Could you check a few things on this model? Use its own coordinates, in mm. Face numbers are marked on the shaded views. A direction names the side the tool comes from. Coordinates: 2 decimals unless noted, no trailing zeros. Order: outer loops, then holes, each group sorted by start corner. A loop starts at its lowest first (then second) coordinate and runs counter-clockwise, first axis right, second up. Notation, with made-up numbers: (-7, 12.25) - (30, 12.25) arc R18 ccw to (30, 26.25) - close; hole circle Ø2 at (-34, 35.5). An arc over 180 degrees is marked (long way). Answer as a JSON object with one key per item and string values. Group by question number.
(1) Which directions (+Z, -Z, +X, -X, +Y, -Y) give clear straight access to the entire face, cutting with the end or side of a thin tool? Please do the marked faces 4, 5 and 6.
(2) Imagine slicing it at B-B, the plane z = -7. Give the number of separate pieces and of enclosed holes in the cut face, and give its area (3 significant figures).
(3) We'd pull the mould along Y, two halves only. Please class the marked faces 1, 2 and 3: pulls with the +Y half, pulls with the -Y half, needs draft (parallel to the pull), parting line crosses it, or undercut.
(4) Please list where these lines run through material, in increasing order: probe 1 along Z at (x, y) = (22, -7); probe 2 along Y at (x, z) = (3.5, -21); probe 3 along Z at (x, y) = (3.5, -31).
(5) Will these pins go through, and if not, where does the flat tip stop? P1, Ø4, axis at y = -43, z = -8, coming from the -X side; P2, Ø5, axis at x = 13.5, z = -18.5, coming from the +Y side; P3, Ø2, axis at x = 0.5, y = -44.5, coming from the -Z side.
(6) Imagine slicing it at A-A, the plane z = -25. Write out the boundary of the cut face in (x, y).
from build123d import *

# Parameters (mm, degrees)
F1_DEPTH  = 17.5
F1_TAPER  = -3.5
F3_DEPTH  = 75
F4_T      = 2
F5_W      = 12.5
F5_H      = 3.5
F6_DEPTH  = 17.5010001
F7_R      = 4
F8_DEPTH  = 31.5
F9_SIZE   = 3
F11_W     = 25
F11_H     = 20
F12_DEPTH = 10


# Not quite as in the source:
# - a shell that OpenCascade refuses in one call is made with other operations: the cavity is built on its own and cut out


with BuildPart() as f1:
    # F0 (on Top) → F1 (new body)
    with BuildSketch(Plane.XY):
        with BuildLine():
            Line((-40.5, -45), (40.5, -45))
            ThreePointArc((40.5, -45), (41.9142135624, -44.4142135624), (42.5, -43))
            Line((42.5, -43), (42.5, 43))
            ThreePointArc((42.5, 43), (41.9142135624, 44.4142135624), (40.5, 45))
            Line((40.5, 45), (-40.5, 45))
            ThreePointArc((-40.5, 45), (-41.9142135624, 44.4142135624), (-42.5, 43))
            Line((-42.5, 43), (-42.5, -43))
            ThreePointArc((-42.5, -43), (-41.9142135624, -44.4142135624), (-40.5, -45))
        make_face()
    extrude(amount=-F1_DEPTH, taper=F1_TAPER)

    # F2 (on Front) → F3 (cut, symmetric)
    with BuildSketch(Plane.XZ):
        Polygon((-20, -17.5), (0, -17.5), (20, -17.5), (12, -9.5), (0, -9.5), (-12, -9.5), align=None)
    extrude(amount=F3_DEPTH, both=True, mode=Mode.SUBTRACT)

    # F4: shell of thickness 2, made by hand


with BuildPart() as f4_core1:
    # F4_t2: copy of F1
    add(f1.part)

    # the walls: a layer under each face that stays
    f4_faces = [f4_core1.faces().sort_by_distance(p)[0] for p in [
        (0, -45.5351729263, -8.75),
        (-42.2926379677, -44.7926379677, -8.75),
        (42.2926379677, -44.7926379677, -8.75),
        (0, 0, 0),
        (-43.0351729263, 0, -8.75),
        (-42.2926379677, 44.7926379677, -8.75),
        (0, 45.5351729263, -8.75),
        (42.2926379677, 44.7926379677, -8.75),
        (43.0351729263, 0, -8.75),
    ]]
    thicken(f4_faces, amount=-F4_T, mode=Mode.SUBTRACT)


with BuildPart() as f1_1:
    add(f1.part)

    # what is left inside the walls is the cavity
    f4_cavity = [f4_core1.part.solids().sort_by_distance(p)[0] for p in [
        (-13.539529, 0, -2.02),
    ]]
    add(f4_cavity, mode=Mode.SUBTRACT)

    # F5 (on Top) → F6 (cut, through all)
    with BuildSketch(Plane.XY):
        with Locations((-32.25, -42.25)):
            Rectangle(F5_W, F5_H)
        with Locations((32.25, -42.25)):
            Rectangle(F5_W, F5_H)
    extrude(amount=-F6_DEPTH, mode=Mode.SUBTRACT)

    # F7 (on Top) → F8 (join)
    with BuildSketch(Plane.XY):
        with Locations((-17, -6)):
            Circle(F7_R)
        with Locations((17, -6)):
            Circle(F7_R)
    extrude(amount=-F8_DEPTH)

    # F9
    f9_edges = [f1_1.edges().sort_by_distance(p)[0] for p in [
        (-21, -6, -31.5),
        (13, -6, -31.5),
    ]]
    chamfer(f9_edges, length=F9_SIZE)

    # F11 (on offset) → F12 (join)
    with BuildSketch(Plane(origin=(0, 0, -23.5), x_dir=(1, 0, 0), z_dir=(0, 0, -1))):
        with Locations((-13, 6)):
            Rectangle(F11_W, F11_H)
        with Locations((13, 6)):
            Rectangle(F11_W, F11_H)
    extrude(amount=-F12_DEPTH)


solid = f1_1.part
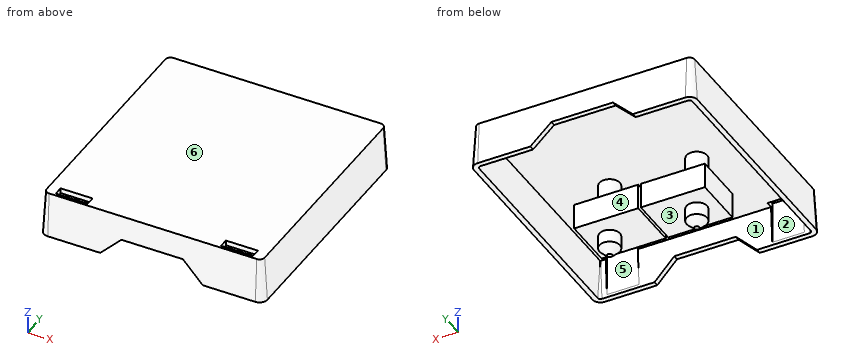
Result set:
{
 "1": {"face 4": "-Z", "face 5": "+Z, -Z", "face 6": "+Z, +X, -X, +Y, -Y"},
 "2": {"separate pieces": "3", "enclosed holes": "1", "area": "773 mm^2"},
 "3": {"face 1": "undercut", "face 2": "undercut", "face 3": "needs draft"},
 "4": {"probe 1": "z = -23.5 to -13.5, -2 to 0", "probe 2": "y = -16 to 4", "probe 3": "z = -2 to 0"},
 "5": {"P1": "stops at x = -43.11", "P2": "stops at y = 4", "P3": "stops at z = -9.5"},
 "6": {"outline": "circle Ø8 at (-17, -6); circle Ø8 at (17, -6)"}
}
